Geometry check sheet. Reference: the model listing, model coordinates, mm. Face numbers are marked on the shaded views. A direction names the side the tool comes from. Round coordinates to 2 decimals unless told otherwise and drop trailing zeros. Write each loop counter-clockwise with the first axis right and the second up, starting at its lowest first coordinate (ties: lowest second). Pieces come first, ordered by that corner, then holes.
Item 1: Cross-section at D-D (z = 3). Enter the section's corners in (x, y), then the cut area to 3 significant figures.
Item 2: Depth check by flat-ended pin: P1, Ø6, axis at x = 75, y = 8, coming from the -Z side. Enter the tip coordinate at first touch or a pass-through.
Item 3: Draft check along Y on the marked faces 1, 2, 3 and 4. Enter one of: pulls with the +Y half, pulls with the -Y half, needs draft (parallel to the pull), parting line crosses it, or undercut.
Item 4: Scan lines: probe 1 along Y at (x, z) = (48, 0.75); probe 2 along Y at (x, z) = (20, 7.75); probe 3 along X at (y, z) = (27, 2.75). Record each from-to range of solid material in increasing order.
Item 5: Access from +Z, -Z, +X, -X, +Y, -Y to the whole of each face (thin tool, end or side, straight path). Record for the marked faces 5 and 6.
Item 6: Cross-section at C-C (x = 39.5). Enter the section's corners in (y, z), then the cut area to 3 significant figures.
Item 7: Cross-section at B-B (y = 19). Enter the section's corners in (x, z), then the cut area to 3 significant figures.
Item 8: Cross-section at A-A (z = 6.5). Enter the section's corners in (x, y).
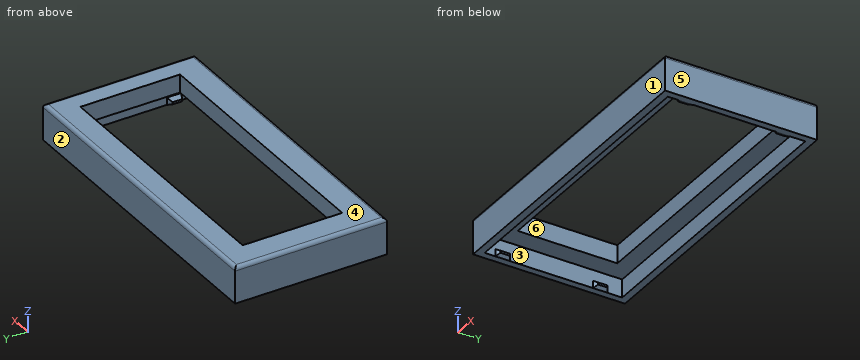
from build123d import *

# Parameters (mm, degrees)
SKETCH_W               = 86
SKETCH_H               = 42
PAD_DEPTH              = 10
FILLET_R               = 1
SKETCH001_W            = 72.65
SKETCH001_H            = 27.54
POCKET_DEPTH           = 10
SKETCH002_W            = 82
SKETCH002_H            = 38
POCKET001_DEPTH        = 5
SKETCH003_W            = 4
SKETCH003_H            = 2
PAD001_DEPTH           = 1.5
PAD001_TAPER           = 25
LINEARPATTERN_COUNT    = 2
LINEARPATTERN_PITCH    = 27
SKETCH004_W            = 4
SKETCH004_H            = 2
PAD002_DEPTH           = 1
PAD002_TAPER           = 35
LINEARPATTERN001_COUNT = 2
LINEARPATTERN001_PITCH = 27


with BuildPart() as part:
    # Sketch → Pad (new body)
    with BuildSketch(Plane.XY):
        with Locations((43, 21)):
            Rectangle(SKETCH_W, SKETCH_H)
    extrude(amount=PAD_DEPTH)

    # Fillet
    fillet_edges = [part.edges().sort_by_distance(p)[0] for p in [
        (43, 42, 10),
        (86, 21, 10),
        (43, 0, 10),
        (0, 21, 10),
    ]]
    fillet(fillet_edges, radius=FILLET_R)

    # Sketch001 (on Face8 of Fillet) → Pocket (cut)
    with BuildSketch(Plane.XY.offset(10)):
        with Locations((43.875, 21.48)):
            Rectangle(SKETCH001_W, SKETCH001_H)
    extrude(amount=-POCKET_DEPTH, mode=Mode.SUBTRACT)

    # Sketch002 (on Face4 of Pocket) → Pocket001 (cut)
    with BuildSketch(Plane(origin=(0, 0, 0), x_dir=(1, 0, 0), z_dir=(0, 0, -1))):
        with Locations((43, -21)):
            Rectangle(SKETCH002_W, SKETCH002_H)
    extrude(amount=-POCKET001_DEPTH, mode=Mode.SUBTRACT)

    # Sketch003 (on Face11 of Pocket001) → Pad001 (join)
    with BuildSketch(Plane(origin=(84, 0, 0), x_dir=(0, -1, 0), z_dir=(-1, 0, 0))):
        with Locations((-7, 1)):
            Rectangle(SKETCH003_W, SKETCH003_H)
    pad001 = extrude(amount=PAD001_DEPTH, taper=PAD001_TAPER)

    # LinearPattern: Pad001 ×2
    with Locations(*[(0, i * LINEARPATTERN_PITCH, 0) for i in range(1, LINEARPATTERN_COUNT)]):
        add(pad001)

    # Sketch004 (on Face15 of LinearPattern) → Pad002 (join)
    with BuildSketch(Plane.YZ.offset(2)):
        with Locations((7, 1)):
            Rectangle(SKETCH004_W, SKETCH004_H)
    pad002 = extrude(amount=PAD002_DEPTH, taper=PAD002_TAPER)

    # LinearPattern001: Pad002 ×2
    with Locations(*[(0, i * LINEARPATTERN001_PITCH, 0) for i in range(1, LINEARPATTERN001_COUNT)]):
        add(pad002)


solid = part.part
Resolved:
1. outline: (0, 0) - (86, 0) - (86, 42) - (0, 42) - close; hole (2, 2) - (84, 2) - (84, 40) - (2, 40) - close
1. area: 496 mm2
2. P1: stops at z = 5
3. face 1: pulls with the -Y half
3. face 2: pulls with the +Y half
3. face 3: undercut
3. face 4: needs draft
4. probe 1: y = 0 to 2, 40 to 42
4. probe 2: y = 0 to 7.71, 35.25 to 42
4. probe 3: x = 0 to 2, 84 to 86
5. face 5: +Z, -Z, +X, +Y, -Y
5. face 6: +Z, -Z
6. outline: (0, 0) - (2, 0) - (2, 5) - (7.71, 5) - (7.71, 10) - (1, 10) arc R1 ccw to (0, 9) - close; (35.25, 5) - (40, 5) - (40, 0) - (42, 0) - (42, 9) arc R1 ccw to (41, 10) - (35.25, 10) - close
6. area: 91.9 mm2
7. outline: (0, 0) - (2, 0) - (2, 5) - (7.55, 5) - (7.55, 10) - (1, 10) arc R1 ccw to (0, 9) - close; (80.2, 5) - (84, 5) - (84, 0) - (86, 0) - (86, 9) arc R1 ccw to (85, 10) - (80.2, 10) - close
7. area: 86.3 mm2
8. outline: (0, 0) - (86, 0) - (86, 42) - (0, 42) - close; hole (7.55, 7.71) - (80.2, 7.71) - (80.2, 35.25) - (7.55, 35.25) - close
